Autodesk Inventor part; units mm, degrees
ref_plane "YZ Plane" through (0, 0, 0) normal (1, 0, 0) x (0, 1, 0)
ref_plane "XZ Plane" through (0, 0, 0) normal (0, 1, 0) x (-1, 0, 0)
ref_plane "XY Plane" through (0, 0, 0) normal (0, 0, 1) x (1, 0, 0)
sketch "Sketch1" plane through (0, 0, 0) normal (0, 1, 0) x (-1, 0, 0)
  line L0 (-30, 12) -> (-34, 12)
  line L1 (-34, 12) -> (-34, 14)
  line L2 (-34, 14) -> (-30, 14)
  line L3 (-30, 14) -> (-30, 16)
  line L4 (-30, 16) -> (-35, 16)
  line L5 (-35, 16) -> (-35, 0)
  line L6 (-35, 0) -> (-30, 0)
  line L7 (-30, 0) -> (-30, 12)
  line L8 (-1, 12) -> (-5, 12)
  line L9 (-5, 12) -> (-5, 0)
  line L10 (-5, 0) -> (0, 0)
  line L11 (0, 0) -> (0, 16)
  line L12 (0, 16) -> (-5, 16)
  line L13 (-5, 16) -> (-5, 14)
  line L14 (-5, 14) -> (-1, 14)
  line L15 (-1, 14) -> (-1, 12)
  line L16 (-35, 0) -> (0, 0)
  line L17 (0, 0) -> (0, -2)
  line L18 (0, -2) -> (-35, -2)
  line L19 (-35, -2) -> (-35, 0)
  line L20 (-35, 16) -> (0, 16)
  line L21 (0, 16) -> (0, -2)
  line L22 (0, -2) -> (-35, -2)
  line L23 (-35, -2) -> (-35, 16)
  line L24 (-35, 16) -> (-30, 0)
  line L25 (-5, 0) -> (0, 16)
  point P0 (-32.5, 8)
  point P1 (-2.5, 8)
  dimension "d0" = 2
extrude "Extrusion1" add sketch "Sketch1" along normal blind 32 contours L16 L10 L17 L18 L19 L6
extrude "Extrusion2" add sketch "Sketch1" against normal blind 2
hole "Hole1" at (32.5, 0, 8) at (2.5, 0, 8) direction (0, -1, 0) diameter 3 depth 8 tip angle 118
sketch "Sketch2" plane through (0, 32, 0) normal (0, 0, 1) x (1, 0, 0)
  line L0 (0, -32) -> (35, -32)
  line L1 (35, -32) -> (35, 0)
  line L2 (0, 0) -> (35, 0)
  line L3 (0, -32) -> (0, 0)
  line L4 (30, -5) -> (30, -27)
  line L5 (30, -27) -> (5, -27)
  line L6 (5, -27) -> (5, -5)
  line L7 (5, -5) -> (30, -5)
  line L8 (25, -22) -> (25, -10)
  line L9 (25, -10) -> (10, -10)
  line L10 (10, -10) -> (10, -22)
  line L11 (10, -22) -> (25, -22)
  line L12 (20, -15) -> (20, -17)
  line L13 (20, -17) -> (15, -17)
  line L14 (15, -17) -> (15, -15)
  line L15 (15, -15) -> (20, -15)
  point P0 (17.5, -5)
  point P1 (17.5, -10)
  point P2 (17.5, -27)
  point P3 (17.5, -22)
  point P4 (17.5, -15)
  point P5 (17.5, -17)
  dimension "d12" = 5
  dimension "d13" = 5
  dimension "d14" = 5
extrude "Extrusion3" cut sketch "Sketch2" against normal blind 10 contours L4 L5 L6 L7 | L12 L13 L14 L15
sketch "Sketch3" plane through (0, 32, 0) normal (0, 0, 1) x (1, 0, 0)
  line L0 (15, -17) -> (15, -15)
  line L1 (20, -15) -> (20, -17)
  line L2 (20, -17) -> (15, -17)
  line L3 (15, -15) -> (20, -15)
  line L4 (15, -17) -> (20, -17)
  line L5 (20, -17) -> (20, -28.4521)
  line L6 (20, -28.4521) -> (15, -28.4521)
  line L7 (15, -28.4521) -> (15, -17)
  line L8 (15, -15) -> (5, -15)
  line L9 (5, -15) -> (5, -17)
  line L10 (5, -17) -> (15, -17)
  line L11 (15, -17) -> (15, -15)
  line L12 (15, -15) -> (20, -15)
  line L13 (20, -15) -> (20, -5)
  line L14 (20, -5) -> (15, -5)
  line L15 (15, -5) -> (15, -15)
  line L16 (20, -15) -> (30, -15)
  line L17 (30, -15) -> (30, -17)
  line L18 (30, -17) -> (20, -17)
  line L19 (20, -17) -> (20, -15)
  line L20 (20, -10) -> (15, -15)
  line L21 (10, -15) -> (15, -17)
  line L22 (15, -17) -> (20, -22)
  line L23 (25, -15) -> (20, -17)
  point P0 (0, -32)
  point P1 (22.5, -16)
  point P2 (17.5, -12.5)
  point P3 (12.5, -16)
  point P4 (17.5, -19.5)
extrude "Extrusion4" add sketch "Sketch3" against normal up to surface (2 mm away) contours L22 L5 L6 L7 | L10 L9 L8 L21 | L2 L5 L22 | L15 L14 L13 L20 | L23 L16 L17 L18
hole "Hole2" at (22.5, 16, 0) at (17.5, 19.5, 0) at (12.5, 16, 0) at (17.5, 12.5, 0) direction (0, 0, -1) diameter 3 depth 8 tip angle 118
properties part number "slide_sensor_base"
Model file for the job. Use its own axes, mm. A direction names the side the tool comes from. Give positions to 0.01 mm unless a question says otherwise; leave off trailing zeros. Write each loop counter-clockwise with the first axis right and the second up, starting at its lowest first coordinate (ties: lowest second). Pieces come first, ordered by that corner, then holes. Notation, with made-up numbers: M 6.25,-37 L 64.25,-37 A22 cw 64.25,-1 Z; hole C 52.5,26 d9. An arc over 180 degrees is marked long. Use a Markdown table: item, result.
1) Cut at A-A (x = 2.5). List the corners of the cut face in (y, z), and give its area (3 significant figures).
Responses:
| item | result |
|---|---|
| outline | M -2,-2 L 32,-2 L 32,0 L 0,0 L 0,6.5 L -2,6.5 Z; M -2,9.5 L 0,9.5 L 0,16 L -2,16 Z |
| area | 94.0 mm2 |
2) Cut at D-D (z = 8). List the corners of the cut face in (x, y).
Responses:
| item | result |
|---|---|
| outline | M 0,-2 L 1,-2 L 1,0 L 0,0 Z; M 4,-2 L 31,-2 L 31,0 L 4,0 Z; M 34,-2 L 35,-2 L 35,0 L 34,0 Z |
3) Tool access for faces 1 (the flat face through (25, 27, -1)), 2 (the flat face through (17.3, 14.8, -2)): list every direction of +Z, -Z, +X, -X, +Y, -Y with a clear straight run to the whole face (end or side of a thin tool).
Responses:
| item | result |
|---|---|
| face 1 | +Z, -Z |
| face 2 | -Z, +X, -X, +Y, -Y |
4) Pin check, flat tip, straight feed: pin 1 (4 mm diameter, centred on x = 17.5, y = 12.5, fed in from +Z). Stop position of the tip, or through.
Responses:
| item | result |
|---|---|
| pin 1 | stops at z = 0 |
5) Drill centre lines: line 1 (Y direction, x = 17.5, z = -0.8); line 2 (Y direction, x = 12.5, z = -0.9); line 3 (X direction, y = 16, z = -0.8). Where is each one in solid material? Low to high. Write a range as from..to.
Responses:
| item | result |
|---|---|
| line 1 | y = -2..11, 14..15, 17..18, 21..32 |
| line 2 | y = -2..5, 10..14.5, 17.5..22, 27..32 |
| line 3 | x = 0..11, 14..15, 20..21, 24..35 |
6) Cut at B-B (y = 12.5). List the corners of the cut face in (x, z), and give its area (3 significant figures).
Responses:
| item | result |
|---|---|
| outline | M 0,-2 L 5,-2 L 5,0 L 0,0 Z; M 10,-2 L 16,-2 L 16,0 L 10,0 Z; M 19,-2 L 25,-2 L 25,0 L 19,0 Z; M 30,-2 L 35,-2 L 35,0 L 30,0 Z |
| area | 44.0 mm2 |
7) Cut at C-C (x = 12.5). List the corners of the cut face in (y, z).
Responses:
| item | result |
|---|---|
| outline | M -2,-2 L 5,-2 L 5,0 L 0,0 L 0,16 L -2,16 Z; M 10,-2 L 14.5,-2 L 14.5,0 L 10,0 Z; M 17.5,-2 L 22,-2 L 22,0 L 17.5,0 Z; M 27,-2 L 32,-2 L 32,0 L 27,0 Z |
8) Pull direction Y, two halves, no side cores. Call faces 3 (the cylindrical face through (1.49, -1.01, 6.89)), 4 (the flat face through (18, -2, 7)), 5 (the flat face through (10, 5, -1)): +Y half, -Y half, draft (parallel to the pull), parting line (faces both ways), or undercut.
Responses:
| item | result |
|---|---|
| face 3 | draft |
| face 4 | -Y half |
| face 5 | undercut |
